Build history of the part. All positions in model axes, mm. A direction names the side the tool comes from. Give positions to 0.01 mm unless a question says otherwise; leave off trailing zeros. Order: outer loops, then holes, each group sorted by start corner. A loop starts at its lowest first (then second) coordinate and runs counter-clockwise, first axis right, second up. Notation, with made-up numbers: (22, 51) - (50, 51) arc R27 cw to (50, 76) - close; hole circle Ø10 at (30.25, 63.5). An arc over 180 degrees is marked (long way). One line per item, written item: value.
```python
from build123d import *

# Parameters (mm, degrees)
IZIM1_W                     = 80
IZIM1_H                     = 32.5
Y_KSEKLIK_EKSTR_ZYON2_DEPTH = 15
IZIM2_W                     = 70
IZIM2_H                     = 13
KES_EKSTR_ZYON1_DEPTH       = 30
IZIM3_W                     = 77
IZIM3_H                     = 3.2
KES_EKSTR_ZYON3_DEPTH       = 30


with BuildPart() as part:
    # Çizim1 → Yükseklik-Ekstrüzyon2 (new body)
    with BuildSketch(Plane(origin=(0, 0, 0), x_dir=(1, 0, 0), z_dir=(0, 1, 0))):
        with Locations((-14.85188748, -6.644700861)):
            Rectangle(IZIM1_W, IZIM1_H)
    extrude(amount=Y_KSEKLIK_EKSTR_ZYON2_DEPTH)

    # Çizim2 → Kes-Ekstrüzyon1 (cut)
    with BuildSketch(Plane.XY.offset(22.894700861)):
        with Locations((-14.85188748, 7.5)):
            Rectangle(IZIM2_W, IZIM2_H)
    extrude(amount=-KES_EKSTR_ZYON1_DEPTH, mode=Mode.SUBTRACT)

    # Çizim3 → Kes-Ekstrüzyon3 (cut)
    with BuildSketch(Plane.XY.offset(22.894700861)):
        with Locations((-14.85188748, 2.6)):
            Rectangle(IZIM3_W, IZIM3_H)
    extrude(amount=-KES_EKSTR_ZYON3_DEPTH, mode=Mode.SUBTRACT)


solid = part.part
```
(1) Pin check, flat tip, straight feed: P1, Ø1.5, axis at x = 13.5, y = 7, coming from the +Z side. Stop position of the tip, or through.
Completed:
P1: z = -7.11
(2) Drill centre lines: line 1 (X direction, y = 11, z = 15.5); line 2 (Y direction, x = 13.5, z = 9.5); line 3 (Y direction, x = 22.5, z = 16). Where is each one in solid material? Low to high.
Completed:
line 1: -54.85 to -49.85, 20.15 to 25.15
line 2: 0 to 1, 14 to 15
line 3: 0 to 1, 4.2 to 15
(3) Slice it at C-C, the plane y = 6. Give the cut face in (x, z).
Completed:
outline: (-54.85, -9.61) - (25.15, -9.61) - (25.15, 22.89) - (20.15, 22.89) - (20.15, -7.11) - (-49.85, -7.11) - (-49.85, 22.89) - (-54.85, 22.89) - close
(4) 3-axis set-ups, long thin cutter, end or side, ignore diameter. For faces 1 (the face through (-15, 1, 8)), 2 (the face through (25.148, 7, 7)): which of +Z, -Z, +X, -X, +Y, -Y reach the whole face in a straight line?
Completed:
face 1: +Z
face 2: +Z, -Z, +X, +Y, -Y
(5) Slice it at A-A, the plane z = 13. Give the cut face in (x, y).
Completed:
outline: (-54.85, 0) - (25.15, 0) - (25.15, 15) - (-54.85, 15) - close; hole (-53.35, 1) - (23.65, 1) - (23.65, 4.2) - (20.15, 4.2) - (20.15, 14) - (-49.85, 14) - (-49.85, 4.2) - (-53.35, 4.2) - close
(6) Pull direction Y, two halves, no side cores. Call faces 3 (the face through (-15, 14, 8)), 4 (the face through (-18, 0.2, 22.895)), 5 (the face through (-15, 15, 6)): +Y half, -Y half, draft (parallel to the pull), parting line (faces both ways), or undercut.
Completed:
face 3: undercut
face 4: draft
face 5: +Y half
(7) Slice it at B-B, the plane x = -39. Give the cut face in (y, z).
Completed:
outline: (0, -9.61) - (15, -9.61) - (15, 22.89) - (14, 22.89) - (14, -7.11) - (1, -7.11) - (1, 22.89) - (0, 22.89) - close
